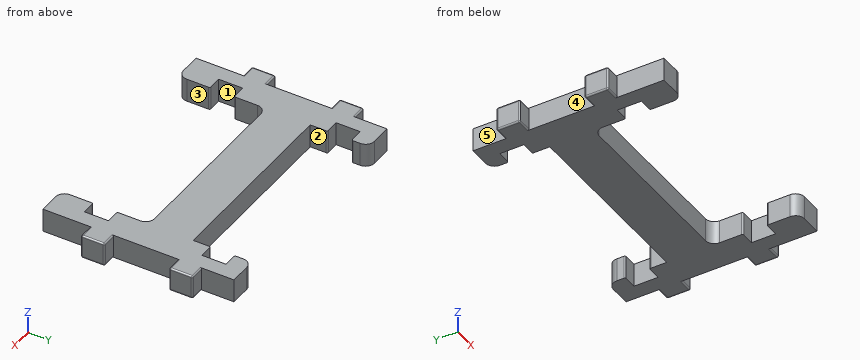
from build123d import *

# Parameters (mm, degrees)
CROQUIS1_W               = 85
CROQUIS1_H               = 65
SALIENTE_EXTRUIR1_DEPTH  = 8
CROQUIS2_W               = 65
CROQUIS2_H               = 20
CORTAR_EXTRUIR1_DEPTH    = 8
CROQUIS3_W               = 65
CROQUIS3_H               = 30
CORTAR_EXTRUIR2_DEPTH    = 8
REDONDEO1_R              = 3
CROQUIS4_W               = 8
CROQUIS4_H               = 8
SALIENTE_EXTRUIR2_DEPTH  = 5
REDONDEO2_R              = 0.5
REDONDEO2_OF_SIMETR_A1_R = 0.5
REDONDEO3_R              = 3
CROQUIS5_W               = 4.8
CROQUIS5_H               = 8.2
CORTAR_EXTRUIR3_DEPTH    = 59.107658703
REDONDEO4_R              = 0.5


with BuildPart() as part:
    # Croquis1 → Saliente-Extruir1 (new body)
    with BuildSketch(Plane.XY):
        Rectangle(CROQUIS1_W, CROQUIS1_H)
    extrude(amount=SALIENTE_EXTRUIR1_DEPTH)

    # Croquis2 → Cortar-Extruir1 (cut)
    with BuildSketch(Plane.XY.offset(8)):
        with Locations((0, 22.5)):
            Rectangle(CROQUIS2_W, CROQUIS2_H)
    extrude(amount=-CORTAR_EXTRUIR1_DEPTH, mode=Mode.SUBTRACT)

    # Croquis3 → Cortar-Extruir2 (cut)
    with BuildSketch(Plane.XY.offset(8)):
        with Locations((0, -17.5)):
            Rectangle(CROQUIS3_W, CROQUIS3_H)
    extrude(amount=-CORTAR_EXTRUIR2_DEPTH, mode=Mode.SUBTRACT)

    # Redondeo1
    redondeo1_edges = [part.edges().sort_by_distance(p)[0] for p in [
        (-32.5, -2.5, 4),
        (32.5, -2.5, 4),
    ]]
    fillet(redondeo1_edges, radius=REDONDEO1_R)

    # Croquis4 → Saliente-Extruir2 (add)
    with BuildSketch(Plane.ZY.offset(42.5)):
        with Locations((4, -12.5)):
            Rectangle(CROQUIS4_W, CROQUIS4_H)
        with Locations((4, 17.5)):
            Rectangle(CROQUIS4_W, CROQUIS4_H)
    saliente_extruir2 = extrude(amount=SALIENTE_EXTRUIR2_DEPTH)

    # Redondeo2
    redondeo2_edges = [part.edges().sort_by_distance(p)[0] for p in [
        (-45, -8.5, 0),
        (-45, -16.5, 0),
        (-45, -16.5, 8),
        (-45, -8.5, 8),
        (-47.5, -12.5, 0),
        (-47.5, -16.5, 4),
        (-47.5, -12.5, 8),
        (-47.5, -8.5, 4),
        (-45, 21.5, 0),
        (-45, 13.5, 0),
        (-45, 13.5, 8),
        (-45, 21.5, 8),
        (-47.5, 17.5, 0),
        (-47.5, 13.5, 4),
        (-47.5, 17.5, 8),
        (-47.5, 21.5, 4),
    ]]
    fillet(redondeo2_edges, radius=REDONDEO2_R)

    # Simetría1: Saliente-Extruir2 across plane
    add(saliente_extruir2.mirror(Plane(origin=(0, 0, 0), x_dir=(0, 0, 1), z_dir=(1, 0, 0))))

    # Redondeo2 of Simetría1
    redondeo2_of_simetr_a1_edges = [part.edges().sort_by_distance(p)[0] for p in [
        (45, -8.5, 0),
        (45, -16.5, 0),
        (45, -16.5, 8),
        (45, -8.5, 8),
        (47.5, -12.5, 0),
        (47.5, -16.5, 4),
        (47.5, -12.5, 8),
        (47.5, -8.5, 4),
        (45, 21.5, 0),
        (45, 13.5, 0),
        (45, 13.5, 8),
        (45, 21.5, 8),
        (47.5, 17.5, 0),
        (47.5, 13.5, 4),
        (47.5, 17.5, 8),
        (47.5, 21.5, 4),
    ]]
    fillet(redondeo2_of_simetr_a1_edges, radius=REDONDEO2_OF_SIMETR_A1_R)

    # Redondeo3
    redondeo3_edges = [part.edges().sort_by_distance(p)[0] for p in [
        (-32.5, 32.5, 4),
        (32.5, 32.5, 4),
        (-32.5, -32.5, 4),
        (32.5, -32.5, 4),
    ]]
    fillet(redondeo3_edges, radius=REDONDEO3_R)

    # Croquis5 → Cortar-Extruir3 (cut, through all)
    with BuildSketch(Plane.XY.offset(8)):
        with Locations((-34.9, 22.5)):
            Rectangle(CROQUIS5_W, CROQUIS5_H)
        with Locations((-34.9, -17.5)):
            Rectangle(CROQUIS5_W, CROQUIS5_H)
        with Locations((34.9, -17.5)):
            Rectangle(CROQUIS5_W, CROQUIS5_H)
        with Locations((34.9, 22.5)):
            Rectangle(CROQUIS5_W, CROQUIS5_H)
    extrude(amount=-CORTAR_EXTRUIR3_DEPTH, mode=Mode.SUBTRACT)

    # Redondeo4
    redondeo4_edges = [part.edges().sort_by_distance(p)[0] for p in [
        (32.5, 26.6, 4),
        (32.5, 18.4, 4),
        (32.5, -13.4, 4),
        (32.5, -21.6, 4),
        (-32.5, -13.4, 4),
        (-32.5, -21.6, 4),
        (-32.5, 26.6, 4),
        (-32.5, 18.4, 4),
    ]]
    fillet(redondeo4_edges, radius=REDONDEO4_R)


solid = part.part
Work out the finished part from the listing and answer in its coordinate system (mm). Face numbers are marked on the shaded views. A direction names the side the tool comes from. Round coordinates to 2 decimals unless told otherwise and drop trailing zeros. Write each loop counter-clockwise with the first axis right and the second up, starting at its lowest first coordinate (ties: lowest second). Pieces come first, ordered by that corner, then holes. Notation, with made-up numbers: M 14,-1.75 L 34,-1.75 A20 cw 34,21.25 Z; hole C -20.5,65 d2. An arc over 180 degrees is marked long. Use a Markdown table: item, result.
1) The part is cut by section D-D on y = 7.5. Give the vertices of the cut face in (x, z).
Taken from the geometry:
| item | result |
|---|---|
| outline | M -42.5,0 L 42.5,0 L 42.5,8 L -42.5,8 Z |
2) The part is cut by section C-C on x = 12.5. Give the vertices of the cut face in (y, z).
Taken from the geometry:
| item | result |
|---|---|
| outline | M -2.5,0 L 12.5,0 L 12.5,8 L -2.5,8 Z |
3) Consider line 1 (Y direction, x = -35.5, z = 2.75); line 2 (X direction, y = 29.5, z = 6.5); line 3 (X direction, y = -19, z = 1). Determine where each line is inside the solid, lowest interval first. Write a range as [from, to].
Taken from the geometry:
| item | result |
|---|---|
| line 1 | y = [-32.5, -21.6], [-13.4, 18.4], [26.6, 32.5] |
| line 2 | x = [-42.5, -32.5], [32.5, 42.5] |
| line 3 | x = [-42.5, -37.3], [37.3, 42.5] |
4) The part is cut by section B-B on y = -27.5. Give the vertices of the cut face in (x, z), plus the area to 3 significant figures.
Taken from the geometry:
| item | result |
|---|---|
| outline | M -42.5,0 L -32.5,0 L -32.5,8 L -42.5,8 Z; M 32.5,0 L 42.5,0 L 42.5,8 L 32.5,8 Z |
| area | 160 mm2 |
5) Flat-ended cylindrical pins translate along their axes: pin 1 (2 mm diameter, centred on x = -45, z = 3, fed in from +Y); pin 2 (1.2 mm diameter, centred on y = 28.5, z = 4, fed in from +X); pin 3 (4 mm diameter, centred on y = 24.5, z = 3, fed in from -X). Find the tip coordinate at first contact, or state that the pin passes through.
Taken from the geometry:
| item | result |
|---|---|
| pin 1 | stops at y = 21.5 |
| pin 2 | stops at x = 42.5 |
| pin 3 | stops at x = -42.5 |
6) The part is cut by section A-A on y = -10. Give the vertices of the cut face in (x, z), plus the area to 3 significant figures.
Taken from the geometry:
| item | result |
|---|---|
| outline | M -47.5,0.5 A0.5 ccw -47,0 L -32.5,0 L -32.5,8 L -47,8 A0.5 ccw -47.5,7.5 Z; M 32.5,0 L 47,0 A0.5 ccw 47.5,0.5 L 47.5,7.5 A0.5 ccw 47,8 L 32.5,8 Z |
| area | 240 mm2 |
7) Determine the mould class of the marked faces 4 and 5 for opening direction Y: pulls with the +Y half, pulls with the -Y half, needs draft (parallel to the pull), parting line crosses it, or undercut.
Taken from the geometry:
| item | result |
|---|---|
| face 4 | undercut |
| face 5 | needs draft |
8) Which of the six approach directions +Z, -Z, +X, -X, +Y, -Y give full straight-line access (tool end or side, diameter ignored) to the marked faces 1, 2 and 3?
Taken from the geometry:
| item | result |
|---|---|
| face 1 | +Z, -Z |
| face 2 | +Z, -Z, +Y |
| face 3 | +Z, -Z, -Y |
